```python
from build123d import *

# Parameters (mm, degrees)
CROQUIS1_W                    = 16
CROQUIS1_H                    = 19
CROQUIS2_R                    = 13
SALIENTE_EXTRUIR1_DEPTH       = 1.5
SALIENTE_EXTRUIR2_START       = 1.5
CROQUIS3_R                    = 13
SALIENTE_EXTRUIR2_DEPTH       = 1.5
TALADRO1_D                    = 3
TALADRO1_CBORE_D              = 18
TALADRO1_CBORE_DEPTH          = 15
DI_METRO_DE_TALADRO_2_0_2_1_D = 2
CORTAR_EXTRUIR1_DEPTH         = 10
CORTAR_EXTRUIR1_DEPTH_BACK    = 6
CROQUIS10_R                   = 1.25
CHAFL_N1_SIZE                 = 0.5


with BuildPart() as part:
    # Croquis1 → Revolución1 (revolve)
    with BuildSketch(Plane(origin=(0, 0, 0), x_dir=(1, 0, 0), z_dir=(0, 1, 0))):
        with Locations((8, 0.635135135)):
            Rectangle(CROQUIS1_W, CROQUIS1_H)
    revolve(axis=Axis((0, 0, -10.135135135), (0, 0, 1)))

    # Croquis2 → Saliente-Extruir1 (add)
    with BuildSketch(Plane.XY.offset(8.864864865)):
        Circle(CROQUIS2_R)
    extrude(amount=SALIENTE_EXTRUIR1_DEPTH)

    # Croquis3 → Saliente-Extruir2 (add)
    with BuildSketch(Plane(origin=(0, 0, -10.135135135), x_dir=(-1, 0, 0), z_dir=(0, 0, -1)).offset(SALIENTE_EXTRUIR2_START)):
        with Locations(Location((0, 0, 0), (0, 0, 180))):
            Circle(CROQUIS3_R)
    extrude(amount=-SALIENTE_EXTRUIR2_DEPTH)

    # Taladro1 (through all)
    with Locations(Plane(origin=(0, 0, -11.635135135), x_dir=(-1, 0, 0), z_dir=(0, 0, -1))):
        with Locations((0, 0)):
            CounterBoreHole(TALADRO1_D / 2, TALADRO1_CBORE_D / 2, TALADRO1_CBORE_DEPTH)

    # Diámetro de taladro Ø2.0 (2)1 (through all)
    with Locations(Plane.XY.offset(10.364864865)):
        with Locations((5.656854249, 5.656854249), (7.72740661, -2.070552361), (2.070552361, -7.72740661), (-5.656854249, -5.656854249), (-7.72740661, 2.070552361), (-2.070552361, 7.72740661)):
            Hole(DI_METRO_DE_TALADRO_2_0_2_1_D / 2)

    # Croquis10 → Cortar-Extruir1 (cut, two sides: drawn at the far end of the back side and taken through both)
    with BuildSketch(Plane(origin=(0, 0, 0), x_dir=(0, 0, -1), z_dir=(1, 0, 0)).offset(-CORTAR_EXTRUIR1_DEPTH_BACK)):
        with Locations(Location((-6.864864865, 0, 0), (0, 0, 180))):
            Circle(CROQUIS10_R)
    extrude(amount=CORTAR_EXTRUIR1_DEPTH + CORTAR_EXTRUIR1_DEPTH_BACK, mode=Mode.SUBTRACT)

    # Chaflán1
    chafl_n1_edges = [part.edges().sort_by_distance(p)[0] for p in [
        (9, 0, -11.635135135),
        (-1.070552361, 7.72740661, 10.364864865),
        (-6.72740661, 2.070552361, 10.364864865),
        (-4.656854249, -5.656854249, 10.364864865),
        (3.070552361, -7.72740661, 10.364864865),
        (8.72740661, -2.070552361, 10.364864865),
        (6.656854249, 5.656854249, 10.364864865),
    ]]
    chamfer(chafl_n1_edges, length=CHAFL_N1_SIZE)


solid = part.part
```
Can you work these out from the model? Positions are in its coordinate system, mm. A direction names the side the tool comes from. Coordinates: 2 decimals unless noted, no trailing zeros. Loops run counter-clockwise (first coordinate to the right, second up) from the corner with the lowest first, then second, coordinate; pieces in that order, holes last. Notation, with made-up numbers: (86.5, 31) -> (137.5, 31) arc R15 cw to (137.5, 37) -> close; hole circle Ø3 at (89.5, -25.75). An arc over 180 degrees is marked (long way). Answer as a JSON object with one key per item and string values.
1) For P1, Ø5, axis at x = -12.5, z = 7.5, coming from the +Y side; P2, Ø2.5, axis at x = 2.07, y = -7.73, coming from the +Z side; P3, Ø2.5, axis at x = -5.66, y = -5.66, coming from the -Z side, each with a flat end and sliding along its axis, tell me the tip position at first contact or that it passes through.
Results:
{"P1": "stops at y = 12.49", "P2": "stops at z = 10.12", "P3": "stops at z = -11.39"}
2) Imagine slicing it at D-D (z = -2.25). Please give me the cut outline in (x, y).
Results:
{"outline": "circle Ø32 at (0, 0); hole circle Ø18 at (0, 0)"}
3) Thinking about a two-plate mould opening in Y: for faces 1 (the face through (1.3, 13.1, -10.135)), 2 (the face through (0, -2, 3.365)), 3 (the face through (10, 0, 7)), 4 (the face through (-10.316, -7.91, 9.604)), which applies, pulls with the +Y half, pulls with the -Y half, needs draft (parallel to the pull), parting line crosses it, or undercut?
Results:
{"face 1": "needs draft", "face 2": "undercut", "face 3": "undercut", "face 4": "parting line crosses it"}
4) Imagine slicing it at C-C (y = -10). Please give me the cut outline in (x, z), then the cut area to 3 significant figures.
Results:
{"outline": "(-12.49, -10.14) -> (-8.31, -10.14) -> (-8.31, -11.64) -> (8.31, -11.64) -> (8.31, -10.14) -> (12.49, -10.14) -> (12.49, 8.86) -> (8.31, 8.86) -> (8.31, 10.36) -> (-8.31, 10.36) -> (-8.31, 8.86) -> (-12.49, 8.86) -> close", "area": "524 mm^2"}
5) For faces 5 (the face through (1.172, 8.923, -3.987)), 6 (the face through (1.3, 13.1, 8.865)), 7 (the face through (3, 0, 10.365)), which set-ups out of +Z, -Z, +X, -X, +Y, -Y let a thin tool reach every point of the face, with its end or its side?
Results:
{"face 5": "-Z", "face 6": "+Z", "face 7": "+Z, +X, -X, +Y, -Y"}
6) Imagine slicing it at A-A (x = 0). Please give me the cut outline in (y, z), then the cut area to 3 significant figures.
Results:
{"outline": "(-16, -10.14) -> (-13, -10.14) -> (-13, -11.64) -> (-9.5, -11.64) -> (-9, -11.14) -> (-9, 3.36) -> (-1.5, 3.36) -> (-1.5, 10.36) -> (-13, 10.36) -> (-13, 8.86) -> (-16, 8.86) -> close; (1.5, 3.36) -> (9, 3.36) -> (9, -11.14) -> (9.5, -11.64) -> (13, -11.64) -> (13, -10.14) -> (16, -10.14) -> (16, 8.86) -> (13, 8.86) -> (13, 10.36) -> (1.5, 10.36) -> close", "area": "395 mm^2"}
7) If I drill on line 1 (Y direction, x = 0, z = -2.5); line 2 (Z direction, x = -4.5, y = -3.5); line 3 (X direction, y = 6.5, z = -2), over which ranges is the centre line in solid material (lowest first)?
Results:
{"line 1": "y = -16 to -9, 9 to 16", "line 2": "z = 3.36 to 10.36", "line 3": "x = -14.62 to -6.22, 6.22 to 14.62"}
